Autodesk Inventor part; units mm, degrees
ref_plane "YZ Plane" through (0, 0, 0) normal (1, 0, 0) x (0, 1, 0)
ref_plane "XZ Plane" through (0, 0, 0) normal (0, 1, 0) x (-1, 0, 0)
ref_plane "XY Plane" through (0, 0, 0) normal (0, 0, 1) x (1, 0, 0)
sketch "Sketch1" plane through (0, 0, 0) normal (1, 0, 0) x (0, 1, 0)
  line L0 (10, 0) -> (10, 150.8357)
  arc A0 (10, 0) -> (24.6447, -35.3553) centre (60, 0) ccw
  line L1 (10, 0) -> (60, 0) construction
  line L2 (24.6447, -35.3553) -> (60, 0) construction
  line L3 (24.6447, -35.3553) -> (0, -35.3553)
  line L4 (10, 150.8357) -> (0, 150.8357)
  line L5 (0, 150.8357) -> (0, -35.3553)
  circle A1 centre (0, 120.8357) radius 10
  point P0 (0, 0)
  dimension "d5" = 50
  dimension "d6" = 45
  dimension "d21" = 20
  dimension "d22" = 30
revolve "Revolution1" add sketch "Sketch1" angle 360 about axis through (0, 0, 150.8357) along (0, 0, -1) picked at (3.0032, 122.282) contours A0 L3 L5 A1 L0 | A1 L5 L4 L0 | A1 L5
fillet "Fillet1" radius 3 1 edges at (0, -10, 150.8357)
sketch "Sketch2" plane through (0, 0, 150.8357) normal (0, 0, 1) x (1, 0, 0)
  point P0 (0, 0)
  point P1 (0, 0)
hole "Hole1" at (0, 0, 150.8357) direction (0, 0, -1) diameter 3 end through all
fillet "Fillet2" radius 50 1 edges at (0, 1.5, -35.3553)
chamfer "Chamfer1" distance 3 angle 45 2 edges at (-24.6447, 0, -35.3553) (24.6447, 0, -35.3553)
ref_plane "Work Plane2" through (0, 10, 0) normal (-1, 0, 0) x (0, 0, 1)
ref_plane "Work Plane1" through (0, 10, 150.8357) normal (0, 1, 0) x (-1, 0, 0)
extrude "Extrusion1" add sketch "Sketch1" along normal blind 30 contours A1 L5 | L5 A1
sketch "Sketch3" plane through (0, 0, 150.8357) normal (0, 0, 1) x (1, 0, 0)
  point P0 (0, 0)
  point P1 (0, 0)
hole "Hole2" at (0, 0, 150.8357) direction (0, 0, -1) diameter 3 end through all
sketch "Sketch5" plane through (30, 0, 120.8357) normal (1, 0, 0) x (0, 0, -1)
  point P0 (120.8357, 0)
  point P1 (0.0315, -0.0065)
sketch "Sketch6" plane through (30, 0, 120.8357) normal (1, 0, 0) x (0, 0, -1)
  point P0 (120.8357, 0)
ref_plane "Work Plane3" through (30, 0, 120.8357) normal (1, 0, 0) x (0, 0, -1)
sketch "Sketch9" plane through (30, 0, 120.8357) normal (1, 0, 0) x (0, 0, -1)
  circle A0 centre (0, 0) radius 4
  point P0 (120.8357, 0)
  dimension "d40" = 8
extrude "Extrusion2" cut sketch "Sketch9" against normal blind 2
equation "\"d5\" = Rbend"
equation "\"d21\" = mainDiameter"
equation "\"d22\" = magnetPosition"
equation "\"d23\" = magnetPosition"
equation "\"d30\" = Thickness"
equation "\"d40\" = magnetDiamter"
equation "\"d41\" = magnetHeight"
equation "\"mainDiameter\" = 20"
equation "\"channelDiameter\" = 1"
equation "\"Rbend\" = 50"
equation "\"BendRadius\" = Thickness"
equation "\"BendReliefWidth\" = Thickness"
equation "\"BendReliefDepth\" = 0.5 * Thickness"
equation "\"CornerReliefSize\" = 4 * Thickness"
equation "\"MinimumRemnant\" = 2 * Thickness"
equation "\"TransitionRadius\" = BendRadius"
equation "\"JacobiRadiusSize\" = BendRadius"
equation "\"GapSize\" = Thickness"
equation "\"magnetPosition\" = 30"
equation "\"magnetDiamter\" = 8"
equation "\"magnetHeight\" = 2"
properties part number "fiberHolder2"
The listing builds one solid part. Answer for the finished solid, in the listing's coordinates (mm). A direction names the side the tool comes from. Coordinates: 2 decimals unless noted, no trailing zeros. Order: outer loops, then holes, each group sorted by start corner. A loop starts at its lowest first (then second) coordinate and runs counter-clockwise, first axis right, second up. Notation, with made-up numbers: M 36.25,-28 L 63.25,-28 A24 ccw 63.25,6 Z; hole C 48.5,6 d4. An arc over 180 degrees is marked long. Answer as a JSON object with one key per item and string values. Group by question number.
1. A tool of negligible diameter and unlimited length cuts with its end or side. For faces 4 (the cylindrical face through (18.12, -9.99, 120.4)), 5 (the cylindrical face through (-9.915, -1.302, 74.953)), 6 (the flat face through (30, 4.3, 121)), from which of +Z, -Z, +X, -X, +Y, -Y can it reach the whole face along a straight path? Write none if from no direction.
2. Section B-B on z = 3.5 is taken. Write down the section's boundary in (x, y), then the cut area to 3 significant figures.
3. Section A-A on z = 62 is taken. Write down the section's boundary in (x, y), then the cut area to 3 significant figures.
4. Straight lines are drawn through the part: line 1 (X direction, y = 0, z = 97); line 2 (Z direction, x = 17, y = 5.5). For each, find the intervals that lie inside material, in ascending order.
5. Flat-ended cylindrical pins translate along their axes: P1, Ø1, axis at x = 13, y = -8, coming from the -Z side; P2, Ø10, axis at y = -0.5, z = 54.5, coming from the -X side; P3, Ø8, axis at x = 13.5, y = -14.5, coming from the +Z side. Find the tip coordinate at first contact, or state that the pin passes through.
6. Determine the mould class of faces 1 (the flat face through (28, 0, 121)), 2 (the flat face through (2, 0, 150.836)), 3 (the cylindrical face through (-0.07, 1.5, 77.82)) for opening direction X: released by +X, released by -X, zero draft, split by the parting line, or undercut.
Values follow:
{
 "1": {"face 4": "+X", "face 5": "none", "face 6": "+Z, -Z, +X, +Y, -Y"},
 "2": {"outline": "C 0,0 d20; hole C 0,0 d3.22", "area": "306 mm2"},
 "3": {"outline": "C 0,0 d20; hole C 0,0 d3", "area": "307 mm2"},
 "4": {"line 1": "-10 to -1.5, 1.5 to 10", "line 2": "-30.18 to -26.92, 112.48 to 129.19"},
 "5": {"P1": "z = -28.15", "P2": "x = -10", "P3": "z = -23.4"},
 "6": {"face 1": "released by +X", "face 2": "zero draft", "face 3": "undercut"}
}
